The listing builds one solid part. Answer for the finished solid, in the listing's coordinates (mm). A direction names the side the tool comes from. Coordinates: 2 decimals unless noted, no trailing zeros. Order: outer loops, then holes, each group sorted by start corner. A loop starts at its lowest first (then second) coordinate and runs counter-clockwise, first axis right, second up. Notation, with made-up numbers: (55.25, -15.5) -> (64.25, -15.5) arc R13 ccw to (64.25, 8.5) -> close; hole circle Ø4 at (-15.5, 57.5). An arc over 180 degrees is marked (long way). One line per question, with ' | ' between items.
from build123d import *

# Parameters (mm, degrees)
F1_DEPTH = 3
F2_R     = 10
F4_DEPTH = 10


with BuildPart() as f1:
    # F0 (on Top) → F1 (new body)
    with BuildSketch(Plane.XY):
        Polygon((55, 50), (-55, 50), (-55, 20), (-90, 20), (-90, -20), (-55, -20), (-55, -50), (55, -50), (55, -20), (90, -20), (90, 20), (55, 20), align=None)
    extrude(amount=F1_DEPTH)

    # F2
    f2_edges = [f1.edges().sort_by_distance(p)[0] for p in [
        (-55, 50, 1.5),
        (55, 50, 1.5),
        (55, -50, 1.5),
        (-55, -50, 1.5),
    ]]
    fillet(f2_edges, radius=F2_R)

    # F3 (on face) → F4 (join)
    with BuildSketch(Plane.XY.offset(3)):
        Polygon((-55, 20), (-90, 20), (-90, -20), (-55, -20), (-55, -18), (-88, -18), (-88, 18), (-55, 18), align=None)
        with BuildLine():
            Line((-55, 40), (-55, 20))
            Line((-55, 20), (-55, 18))
            Line((-55, 18), (-53, 18))
            Line((-53, 18), (-53, 38))
            ThreePointArc((-53, 38), (-50.071068, 45.071068), (-43, 48))
            Line((-43, 48), (43, 48))
            ThreePointArc((43, 48), (50.071068, 45.071068), (53, 38))
            Line((53, 38), (53, 18))
            Line((53, 18), (55, 18))
            Line((55, 18), (55, 20))
            Line((55, 20), (55, 40))
            ThreePointArc((55, 40), (52.071068, 47.071068), (45, 50))
            Line((45, 50), (-45, 50))
            ThreePointArc((-45, 50), (-52.071068, 47.071068), (-55, 40))
        make_face()
        with BuildLine():
            Line((-55, -18), (-55, -20))
            Line((-55, -20), (-55, -40))
            ThreePointArc((-55, -40), (-52.071068, -47.071068), (-45, -50))
            Line((-45, -50), (45, -50))
            ThreePointArc((45, -50), (52.071068, -47.071068), (55, -40))
            Line((55, -40), (55, -20))
            Line((55, -20), (55, -18))
            Line((55, -18), (53, -18))
            Line((53, -18), (53, -38))
            ThreePointArc((53, -38), (50.071068, -45.071068), (43, -48))
            Line((43, -48), (-43, -48))
            ThreePointArc((-43, -48), (-50.071068, -45.071068), (-53, -38))
            Line((-53, -38), (-53, -18))
            Line((-53, -18), (-55, -18))
        make_face()
        Polygon((90, 20), (55, 20), (55, 18), (88, 18), (88, -18), (55, -18), (55, -20), (90, -20), align=None)
    extrude(amount=F4_DEPTH)


solid = f1.part
Item 1: Each of these flat-tipped pins is pushed along its axis until it touches: pin 1 Ø2 at (y, z) = (27, 4.5) entering from -X; pin 2 Ø3 at (y, z) = (-23.5, 10) entering from +X; pin 3 Ø6.5 at (x, z) = (81, 9) entering from +Y. Where does it stop, or does it pass through?
Computed values:
pin 1: stops at x = -55 | pin 2: stops at x = 55 | pin 3: stops at y = 20
Item 2: For faces 1 (the face through (71, -18, 8)), 2 (the face through (55, -30, 6)), 3 (the face through (-55, 30, 6)), 4 (the face through (55, 30, 6)), determine the directions among +Z, -Z, +X, -X, +Y, -Y from which every point of the face is accessible in a straight line to the end or side of a thin tool.
Computed values:
face 1: +Z | face 2: +Z, -Z, +X, -Y | face 3: +Z, -Z, -X, +Y | face 4: +Z, -Z, +X, +Y
Item 3: Determine the mould class of faces 5 (the face through (53, -28, 8)), 6 (the face through (1, -48, 8)), 7 (the face through (-1, -50, 6)), 8 (the face through (-90, 0, 6)) for opening direction X: pulls with the +X half, pulls with the -X half, needs draft (parallel to the pull), parting line crosses it, or undercut.
Computed values:
face 5: undercut | face 6: undercut | face 7: needs draft | face 8: pulls with the -X half
Item 4: Find the intervals of material crossed by L1, parallel to X at y = 34.5, z = 10.25; L2, parallel to Y at x = -72.5, z = 8.5; L3, parallel to Y at x = 37, z = 3.5, in increasing order.
Computed values:
L1: x = -55 to -53, 53 to 55 | L2: y = -20 to -18, 18 to 20 | L3: y = -50 to -48, 48 to 50
Item 5: Section B-B, the plane x = -31 is taken. Give the vertices of the cut face in (y, z), plus the area to 3 significant figures.
Computed values:
outline: (-50, 0) -> (50, 0) -> (50, 13) -> (48, 13) -> (48, 3) -> (-48, 3) -> (-48, 13) -> (-50, 13) -> close | area: 340 mm^2
Item 6: Section A-A, the plane y = 1.5 is taken. Give the vertices of the cut face in (x, z).
Computed values:
outline: (-90, 0) -> (90, 0) -> (90, 13) -> (88, 13) -> (88, 3) -> (-88, 3) -> (-88, 13) -> (-90, 13) -> close
